```python
from build123d import *

# Parameters (mm, degrees)
SKETCH1_R                 = 3.175
BOSS_EXTRUDE1_DEPTH       = 149.86
F_8_32_TAPPED_HOLE1_D     = 3.4544
F_8_32_TAPPED_HOLE1_DEPTH = 12.7
F_8_32_TAPPED_HOLE1_TIP   = 1.037806461
F_8_32_TAPPED_HOLE2_D     = 3.4544
F_8_32_TAPPED_HOLE2_DEPTH = 15.0876
F_8_32_TAPPED_HOLE2_TIP   = 1.037806461
SKETCH6_R                 = 1.1303
CUT_EXTRUDE1_DEPTH        = 4.175
CUT_EXTRUDE1_DEPTH_BACK   = 4.175


with BuildPart() as part:
    # Sketch1 → Boss-Extrude1 (new body)
    with BuildSketch(Plane(origin=(0, 0, 0), x_dir=(1, 0, 0), z_dir=(0, 1, 0))):
        Circle(SKETCH1_R)
    extrude(amount=BOSS_EXTRUDE1_DEPTH)

    # #8-32 Tapped Hole1
    with Locations(Plane(origin=(0, 0, 0), x_dir=(-1, 0, 0), z_dir=(0, -1, 0))):
        with Locations((0, 0)):
            Hole(F_8_32_TAPPED_HOLE1_D / 2, depth=F_8_32_TAPPED_HOLE1_DEPTH)
            with Locations((0, 0, -(F_8_32_TAPPED_HOLE1_DEPTH + F_8_32_TAPPED_HOLE1_TIP / 2))):  # 118° drill point
                Cone(0, F_8_32_TAPPED_HOLE1_D / 2, F_8_32_TAPPED_HOLE1_TIP, mode=Mode.SUBTRACT)

    # #8-32 Tapped Hole2
    with Locations(Plane(origin=(0, 149.86, 0), x_dir=(1, 0, 0), z_dir=(0, 1, 0))):
        with Locations((0, 0)):
            Hole(F_8_32_TAPPED_HOLE2_D / 2, depth=F_8_32_TAPPED_HOLE2_DEPTH)
            with Locations((0, 0, -(F_8_32_TAPPED_HOLE2_DEPTH + F_8_32_TAPPED_HOLE2_TIP / 2))):  # 118° drill point
                Cone(0, F_8_32_TAPPED_HOLE2_D / 2, F_8_32_TAPPED_HOLE2_TIP, mode=Mode.SUBTRACT)

    # Sketch6 → Cut-Extrude1 (cut, two sides)
    with BuildSketch(Plane.XY) as cut_extrude1_sk:
        with Locations((0, 134.62)):
            Circle(SKETCH6_R)
        with Locations((0, 15.24)):
            Circle(SKETCH6_R)
    extrude(amount=CUT_EXTRUDE1_DEPTH, mode=Mode.SUBTRACT)
    extrude(cut_extrude1_sk.sketch, amount=-CUT_EXTRUDE1_DEPTH_BACK, mode=Mode.SUBTRACT)


solid = part.part
```
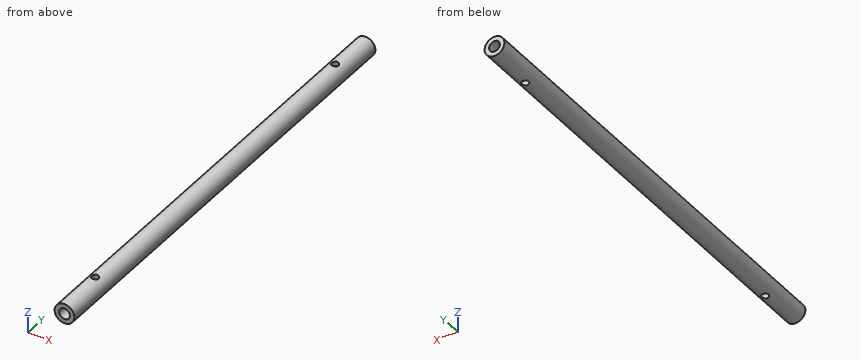
Verification items for the finished model (mm, model axes). Round coordinates to 2 decimals unless told otherwise and drop trailing zeros. Order: outer loops, then holes, each group sorted by start corner. A loop starts at its lowest first (then second) coordinate and runs counter-clockwise, first axis right, second up.
1) Cross-section at A-A, the plane y = 83.5. Record the cut outline in (x, z) (3 decimals).
Geometry says:
outline: circle Ø6.35 at (0, 0)
2) Material ranges on line 1 (Y direction, x = 0.25, z = 2.25); line 2 (Z direction, x = 0, y = 8) (3 decimals); line 3 (Y direction, x = 0, z = 0), recorded low to high.
Geometry says:
line 1: y = 0 to 14.14, 16.34 to 133.52, 135.72 to 149.86
line 2: z = -3.175 to -1.727, 1.727 to 3.175
line 3: y = 13.74 to 14.11, 16.37 to 133.49
3) Depth check by flat-ended pin: pin 1 (1.5 mm diameter, centred on y = 86.5, z = -1.5, fed in from -X); pin 2 (2 mm diameter, centred on x = 0, y = 134.62, fed in from -Z); pin 3 (2 mm diameter, centred on x = 0, z = 0, fed in from -Y); pin 4 (3 mm diameter, centred on x = 0, z = 0, fed in from -Y). Enter the tip coordinate at first touch or a pass-through.
Geometry says:
pin 1: stops at x = -3.09
pin 2: passes through
pin 3: stops at y = 13.14
pin 4: stops at y = 12.84
4) Cross-section at B-B, the plane y = 11. Record the cut outline in (x, z) (3 decimals).
Geometry says:
outline: circle Ø6.35 at (0, 0); hole circle Ø3.454 at (0, 0)
